Geometry: final body of the model. Coordinates: model frame, mm. Give positions to 0.01 mm unless a question says otherwise; leave off trailing zeros. Order: outer loops, then holes, each group sorted by start corner. A loop starts at its lowest first (then second) coordinate and runs counter-clockwise, first axis right, second up. Notation, with made-up numbers: (34, 20.25) -> (73, 20.25) arc R23 cw to (73, 29.25) -> close; hole circle Ø6 at (-11.75, 25). An arc over 180 degrees is marked (long way). One line per question, with ' | ' between items.
Autodesk Inventor part; units mm, degrees
ref_plane "YZ Plane" through (0, 0, 0) normal (1, 0, 0) x (0, 1, 0)
ref_plane "XZ Plane" through (0, 0, 0) normal (0, 1, 0) x (-1, 0, 0)
ref_plane "XY Plane" through (0, 0, 0) normal (0, 0, 1) x (1, 0, 0)
sketch "Sketch1" plane through (0, 0, 0) normal (0, 1, 0) x (-1, 0, 0)
  line L0 (0, 0) -> (134.38, 0)
  line L1 (134.38, 0) -> (67.2135, 125.8908)
  line L2 (67.2135, 125.8908) -> (0, 0)
  circle A0 centre (8.2321, 4.6489) radius 1
  circle A1 centre (126.1421, 4.6489) radius 1
  circle A2 centre (67.2131, 115.5697) radius 1
extrude "Extrusion1" add sketch "Sketch1" along normal blind 2
properties part number "bcc_pcb"
1) Contact query for flat-ended pins moving along their axis: pin 1 Ø1.2 at (x, z) = (-8.23, 4.65) entering from +Y; pin 2 Ø2.5 at (x, z) = (-126.14, 4.65) entering from +Y. Output: stop coordinate, or through.
Check result:
pin 1: passes through | pin 2: stops at y = 2
2) Section B-B on x = -25.5. Return loops of the section in (y, z), plus the area to 3 significant figures.
Check result:
outline: (0, 0) -> (2, 0) -> (2, 47.76) -> (0, 47.76) -> close | area: 95.5 mm^2
3) Material intervals for probe 1 along X at (y, z) = (0.3, 28); probe 2 along Z at (x, y) = (-69, 0.1); probe 3 along X at (y, z) = (1.2, 72), sorted ascending. Write a range as from..to.
Check result:
probe 1: x = -119.44..-14.95 | probe 2: z = 0..122.54 | probe 3: x = -95.97..-38.44
4) Section A-A on y = 1.15. Return loops of the section in (x, z).
Check result:
outline: (-134.38, 0) -> (0, 0) -> (-67.21, 125.89) -> close; hole circle Ø2 at (-126.14, 4.65); hole circle Ø2 at (-67.21, 115.57); hole circle Ø2 at (-8.23, 4.65)
5) Section C-C on z = 19. Return loops of the section in (x, y), plus the area to 3 significant figures.
Check result:
outline: (-124.24, 0) -> (-10.14, 0) -> (-10.14, 2) -> (-124.24, 2) -> close | area: 228 mm^2
